from build123d import *

# Parameters (mm, degrees)
SKETCH_1_W               = 80
SKETCH_1_H               = 73
SKETCH_1_R               = 5
EXTRUDE_1_DEPTH          = 2
PATTERN_CIRCULAR_1_COUNT = 4
FILLET_1_R               = 10
MM_TRANSITIONAL_1_D      = 3
MM_TRANSITIONAL_2_D      = 3


with BuildPart() as part:
    # 草图1 → 凸台-拉伸1 (new body)
    with BuildSketch(Plane(origin=(0, 0, -1.3), x_dir=(-1, 0, 0), z_dir=(0, 0, -1))):
        with Locations((0, 3.5)):
            Rectangle(SKETCH_1_W, SKETCH_1_H)
        Circle(SKETCH_1_R, mode=Mode.SUBTRACT)
    extrude(amount=EXTRUDE_1_DEPTH)

    # 草图3 → 打孔尺寸(%根据十字)槽沉头自攻螺钉的类型1 (revolve, cut)
    with BuildSketch(Plane(origin=(11, 0, -1.3), x_dir=(0, -1, 0), z_dir=(1, 0, 0))):
        Polygon((0, 0), (0, 5.431333959), (1.55, 4.5), (1.55, 1.6), (3.15, 0), align=None)
    hole_wizard_1 = revolve(axis=Axis((11, 0, 5.05), (0, 0, -1)), mode=Mode.SUBTRACT)

    # 阵列(圆周)1: 打孔尺寸(%根据十字)槽沉头自攻螺钉的类型1 ×4 about axis
    pattern_circular_1_axis = Axis((0, 0, 0), (0, 0, 1))
    for i in range(1, PATTERN_CIRCULAR_1_COUNT):
        add(hole_wizard_1.rotate(pattern_circular_1_axis, i * 360 / PATTERN_CIRCULAR_1_COUNT), mode=Mode.SUBTRACT)

    # 圆角1
    fillet_1_edges = [part.edges().sort_by_distance(p)[0] for p in [
        (40, 40, -2.3),
        (-40, 40, -2.3),
    ]]
    fillet(fillet_1_edges, radius=FILLET_1_R)

    # 大小mm Transitional 暗销孔1 (through all)
    with Locations(Plane(origin=(0, 0, -3.3), x_dir=(-1, 0, 0), z_dir=(0, 0, -1))):
        with Locations((-14.60943136, -22), (18, -22)):
            Hole(MM_TRANSITIONAL_1_D / 2)

    # 大小mm Transitional 暗销孔2 (through all)
    with Locations(Plane.XY.offset(-1.3)):
        with Locations((-20.391925208, -9.508910889), (-22.5, 0), (-20.391925208, 9.508910889), (20.391925208, -9.508910889), (22.5, 0), (20.391925208, 9.508910889)):
            Hole(MM_TRANSITIONAL_2_D / 2)


solid = part.part
Input: part model. Units: mm. Frame: model coordinates. Coordinates: 2 decimals unless noted, no trailing zeros. Order: outer loops, then holes, each group sorted by start corner. A loop starts at its lowest first (then second) coordinate and runs counter-clockwise, first axis right, second up. Notation, with made-up numbers: M -38,89.25 L -34,89.25 A28 cw -34,118.25 Z; hole C -40,-3 d3. An arc over 180 degrees is marked long. Write item = value, one per line. Start each with the question number.
(1) Section A-A on x = -18. Output: boundary loops of the cut face in (y, z).
(2) First-contact query: P1, Ø4, axis at x = 0, y = 11, coming from the +Z side; P2, Ø5, axis at x = -11, y = 0, coming from the +Z side. Flat tips, straight axial feed; report the tip coordinate or a pass-through.
(3) Section C-C on x = 11. Output: boundary loops of the cut face in (y, z), and give its area (3 significant figures).
(4) Pull-direction query (X, two-part tool) for faces 1 (the cylindrical face through (37.15, 36.99, -2.31)), 2 (the cylindrical face through (14.414, -20.513, -2.286)), 3 (the flat face through (9, 4, -3.3)); classes: released by +X, released by -X, zero draft, split by the parting line, or undercut.
(5) Section D-D on x = 35. Output: boundary loops of the cut face in (y, z).
(6) Line query: line 1 along Y through (x, z) = (0, -3.05); line 2 along X through (y, z) = (-10.5, -2.1); line 3 along X through (y, z) = (-21, -2.25). Output: solid intervals per line, ascending. Write a range as [from, to].
(7) Section B-B on z = -1.9. Give the number of separate pieces and of enclosed holes in the cut face, and give its area (3 significant figures).
Result set:
q1.outline = M -33,-3.3 L -23.5,-3.3 L -23.5,-1.3 L -33,-1.3 Z; M -20.5,-3.3 L 40,-3.3 L 40,-1.3 L -20.5,-1.3 Z
q2.P1 = -2.45
q2.P2 = -1.95
q3.outline = M -33,-3.3 L -1.55,-3.3 L -1.55,-2.9 L -3.15,-1.3 L -33,-1.3 Z; M 1.55,-3.3 L 40,-3.3 L 40,-1.3 L 3.15,-1.3 L 1.55,-2.9 Z
q3.area = 137 mm²
q4.face_1 = released by +X
q4.face_2 = undercut
q4.face_3 = zero draft
q5.outline = M -33,-3.3 L 38.66,-3.3 L 38.66,-1.3 L -33,-1.3 Z
q6.line_1 = [-33, -12.55], [-9.45, -5], [5, 9.45], [12.55, 40]
q6.line_2 = [-40, -21.52], [-19.27, -2.3], [2.3, 19.27], [21.52, 40]
q6.line_3 = [-40, -19.12], [-16.88, 13.49], [15.73, 40]
q7.separate_pieces = 1
q7.enclosed_holes = 13
q7.area = 5,580 mm²
